from build123d import *

# Parameters (mm, degrees)
SKETCH1_R           = 12.5
BOSS_EXTRUDE1_DEPTH = 52.5
CHAMFER1_SIZE       = 1


with BuildPart() as part:
    # Sketch1 → Boss-Extrude1 (new body, symmetric)
    with BuildSketch(Plane.XY):
        Circle(SKETCH1_R)
    extrude(amount=BOSS_EXTRUDE1_DEPTH, both=True)

    # Chamfer1
    chamfer1_edges = [part.edges().sort_by_distance(p)[0] for p in [
        (-12.5, 0, -52.5),
        (-12.5, 0, 52.5),
    ]]
    chamfer(chamfer1_edges, length=CHAMFER1_SIZE)

    # Sketch4 → Tap Drill for M6 Tap1 (revolve, cut)
    with BuildSketch(Plane(origin=(0, 0, 52.5), x_dir=(0, -1, 0), z_dir=(1, 0, 0))):
        Polygon((0, 0), (0, 14.502151548), (2.5, 13), (2.5, 0), align=None)
    tap_drill_for_m6_tap1 = revolve(axis=Axis((0, 0, 58.85), (0, 0, -1)), mode=Mode.SUBTRACT)

    # Mirror1: Tap Drill for M6 Tap1 across plane
    add(tap_drill_for_m6_tap1.mirror(Plane.XY), mode=Mode.SUBTRACT)


solid = part.part
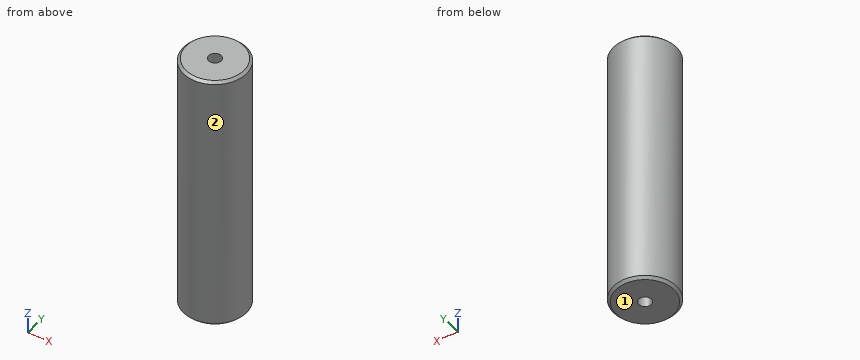
Geometry: final body of the model. Coordinates: model frame, mm. Face numbers are marked on the shaded views. Give positions to 0.01 mm unless a question says otherwise; leave off trailing zeros. Order: outer loops, then holes, each group sorted by start corner. A loop starts at its lowest first (then second) coordinate and runs counter-clockwise, first axis right, second up. Notation, with made-up numbers: (73, 87.25) - (103, 87.25) arc R19 ccw to (103, 109.25) - close; hole circle Ø3 at (-15.75, 2.25). An arc over 180 degrees is marked (long way). Use CSV: the item, a comma, the result in double quotes.
1. Mould query, pull axis X, two halves, no side actions, for the marked faces 1 and 2. Classes: +X half, -X half, draft (parallel to the pull), parting line (faces both ways), or undercut.
Answers below:
face 1,"draft"
face 2,"parting line"
2. Section query B-B (z = 44). Output: boundary loops of the cut face in (x, y).
Answers below:
outline,"circle Ø25 at (0, 0); hole circle Ø5 at (0, 0)"
3. Contact query for flat-ended pins moving along their axis: pin 1 (3 mm diameter, centred on y = 7.5, z = 36, fed in from -X); pin 2 (4 mm diameter, centred on x = 0, y = 0, fed in from -Z); pin 3 (12 mm diameter, centred on x = -9, z = -41, fed in from -Y). Output: stop coordinate, or through.
Answers below:
pin 1,"x = -10.97"
pin 2,"z = -39.2"
pin 3,"y = -12.13"
4. Section query A-A (z = 4.5). Output: boundary loops of the cut face in (x, y).
Answers below:
outline,"circle Ø25 at (0, 0)"
5. Material intervals for line 1 along Y through (x, z) = (0, -42.5); line 2 along Y through (x, z) = (-0.5, 36); line 3 along Y through (x, z) = (-0.5, 44), sorted ascending. Write a range as from..to.
Answers below:
line 1,"-12.5..-2.5, 2.5..12.5"
line 2,"-12.49..12.49"
line 3,"-12.49..-2.45, 2.45..12.49"
